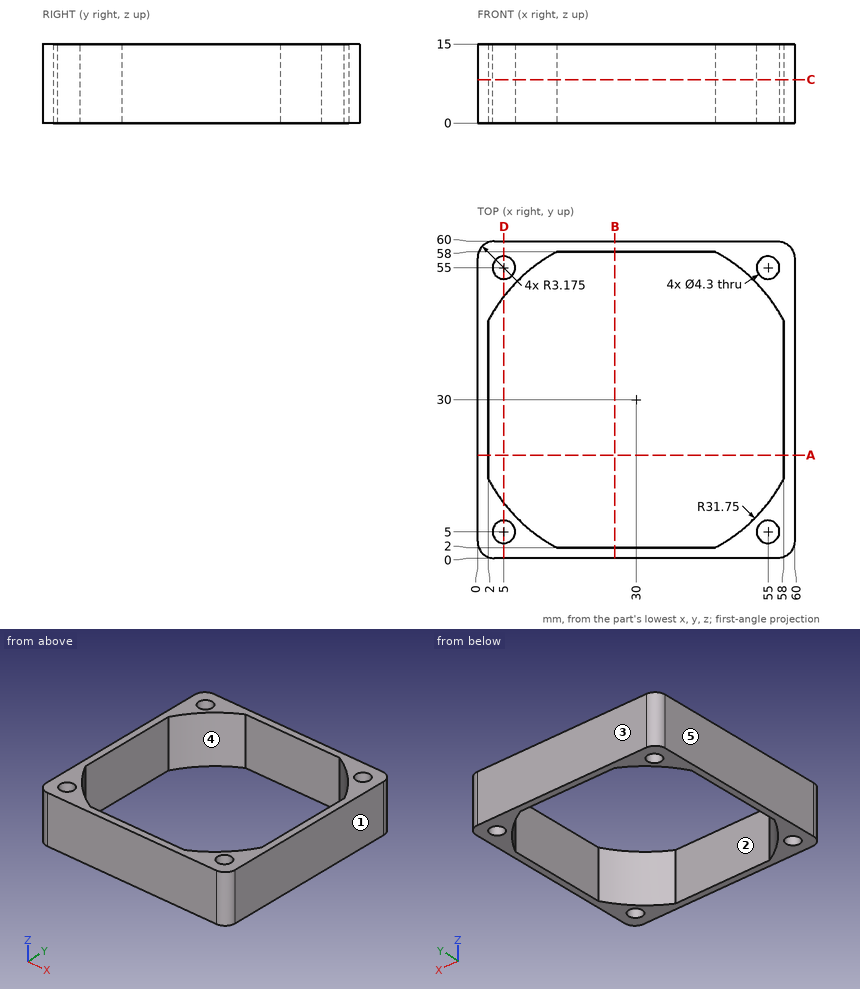
Could you check a few things on this drawing? It's one solid part, dimensions in mm from its lowest x, y, z. A direction names the side the tool comes from. Round coordinates to 2 decimals unless told otherwise and drop trailing zeros. Order: outer loops, then holes, each group sorted by start corner. A loop starts at its lowest first (then second) coordinate and runs counter-clockwise, first axis right, second up. Notation, with made-up numbers: M 55.25,17 L 112.25,17 A16 cw 112.25,22 Z; hole C 3.25,54.25 d7. An arc over 180 degrees is marked long. Return JSON: item names as keys, results as strings. Group by question number.
1. Please list where these lines run through material, in increasing order: probe 1 along Y at (x, z) = (56, 1.25); probe 2 along Y at (x, z) = (5, 5.75); probe 3 along Y at (x, z) = (37.5, 5.5).
2. If we section it at C-C on z = 8.25: List the corners of the cut face in (x, y) for me (3 decimals).
3. If we section it at D-D on x = 5: List the corners of the cut face in (y, z) for me.
4. If we section it at A-A on y = 19.5: List the corners of the cut face in (x, z) for me.
5. I'm going to push flat-ended pins straight in: pin 1 Ø7.5 at (y, z) = (30, 10) entering from -X; pin 2 Ø4 at (x, y) = (55, 5) entering from +Z. Where does each tip first touch, or does it pass through?
6. If we mould it in two halves opening along Y, with no side actions, what happens to the marked faces 1, 2 and 3? For each: pulls with the +Y half, pulls with the -Y half, needs draft (parallel to the pull), parting line crosses it, or undercut.
7. On a 3-axis mill with a long thin cutter (end or side, diameter ignored), from which of +Z, -Z, +X, -X, +Y, -Y can I reach the whole of each face in a straight line? I mean the marked faces 4 and 5. Say none if no direction works.
Reply:
{
 "1": {"probe 1": "0 to 3.1, 6.9 to 11.78, 48.22 to 53.1, 56.9 to 60", "probe 2": "0 to 2.85, 7.15 to 10.43, 49.57 to 52.85, 57.15 to 60", "probe 3": "0 to 2, 58 to 60"},
 "2": {"outline": "M 0,3.175 A3.175 ccw 3.175,0 L 56.825,0 A3.175 ccw 60,3.175 L 60,56.825 A3.175 ccw 56.825,60 L 3.175,60 A3.175 ccw 0,56.825 Z; hole M 2,15.031 A31.75 ccw 15.031,2 L 44.969,2 A31.75 ccw 58,15.031 L 58,44.969 A31.75 ccw 44.969,58 L 15.031,58 A31.75 ccw 2,44.969 Z; hole C 5,5 d4.3; hole C 5,55 d4.3; hole C 55,5 d4.3; hole C 55,55 d4.3"},
 "3": {"outline": "M 0,0 L 2.85,0 L 2.85,15 L 0,15 Z; M 7.15,0 L 10.43,0 L 10.43,15 L 7.15,15 Z; M 49.57,0 L 52.85,0 L 52.85,15 L 49.57,15 Z; M 57.15,0 L 60,0 L 60,15 L 57.15,15 Z"},
 "4": {"outline": "M 0,0 L 2,0 L 2,15 L 0,15 Z; M 58,0 L 60,0 L 60,15 L 58,15 Z"},
 "5": {"pin 1": "x = 0", "pin 2": "through"},
 "6": {"face 1": "needs draft", "face 2": "undercut", "face 3": "pulls with the +Y half"},
 "7": {"face 4": "+Z, -Z", "face 5": "+Z, -Z, -X, +Y, -Y"}
}
